from build123d import *

# Parameters (mm, degrees)
SKETCH2_R           = 14.2875
SKETCH2_R_2         = 3.556
BOSS_EXTRUDE1_DEPTH = 6.35


with BuildPart() as part:
    # Sketch2 → Boss-Extrude1 (new body)
    with BuildSketch(Plane(origin=(0, 0, 0), x_dir=(0, 0, -1), z_dir=(1, 0, 0))):
        with BuildLine():
            Line((-165.1, 34.925), (-80.596664787, 34.925))
            ThreePointArc((-80.596664787, 34.925), (-75.736585196, 33.958270063), (-71.616408666, 31.205256121))
            Line((-71.616408666, 31.205256121), (-20.205576272, -20.205576272))
            ThreePointArc((-20.205576272, -20.205576272), (-17.495774254, -22.592664922), (-14.50653847, -24.618914814))
            Line((-14.50653847, -24.618914814), (68.578013642, -73.575957012))
            ThreePointArc((68.578013642, -73.575957012), (78.454344121, -74.862548761), (86.221769537, -68.628422964))
            Line((86.221769537, -68.628422964), (133.536181692, 14.57458872))
            ThreePointArc((133.536181692, 14.57458872), (135.152284875, 21.909694343), (132.341634936, 28.875023547))
            Line((132.341634936, 28.875023547), (22.151863474, 164.100639036))
            ThreePointArc((22.151863474, 164.100639036), (-9.579695356, 172.971368128), (-28.575, 146.05))
            Line((-28.575, 146.05), (-33.807973228, 116.372334072))
            ThreePointArc((-33.807973228, 116.372334072), (-35.979801138, 112.610617786), (-40.061502459, 111.125))
            Line((-40.061502459, 111.125), (-88.9, 111.125))
            ThreePointArc((-88.9, 111.125), (-91.14506403, 110.19506403), (-92.075, 107.95))
            Line((-92.075, 107.95), (-92.075, 66.675))
            ThreePointArc((-92.075, 66.675), (-93.934871939, 62.184871939), (-98.425, 60.325))
            Line((-98.425, 60.325), (-165.1, 60.325))
            ThreePointArc((-165.1, 60.325), (-167.34506403, 59.39506403), (-168.275, 57.15))
            Line((-168.275, 57.15), (-168.275, 38.1))
            ThreePointArc((-168.275, 38.1), (-167.34506403, 35.85493597), (-165.1, 34.925))
        make_face()
        with Locations((0, 146.05)):
            Circle(SKETCH2_R, mode=Mode.SUBTRACT)
        Circle(SKETCH2_R, mode=Mode.SUBTRACT)
        with Locations((-53.975, 47.625)):
            Circle(SKETCH2_R_2, mode=Mode.SUBTRACT)
        with Locations((-79.375, 47.625)):
            Circle(SKETCH2_R_2, mode=Mode.SUBTRACT)
        with Locations((-104.775, 47.625)):
            Circle(SKETCH2_R_2, mode=Mode.SUBTRACT)
        with Locations((-130.175, 47.625)):
            Circle(SKETCH2_R_2, mode=Mode.SUBTRACT)
        with Locations((-155.575, 47.625)):
            Circle(SKETCH2_R_2, mode=Mode.SUBTRACT)
        with Locations((100.217738322, 10.071728166)):
            Circle(SKETCH2_R, mode=Mode.SUBTRACT)
        with Locations((-79.375, 73.025)):
            Circle(SKETCH2_R_2, mode=Mode.SUBTRACT)
        with Locations((-79.375, 98.425)):
            Circle(SKETCH2_R_2, mode=Mode.SUBTRACT)
        with BuildLine():
            Line((108.137843951, 33.631444269), (108.400752916, 34.22590106))
            ThreePointArc((108.400752916, 34.22590106), (111.416042328, 35.39192926), (112.582070528, 32.376639848))
            Line((112.582070528, 32.376639848), (112.319161563, 31.782183057))
            ThreePointArc((112.319161563, 31.782183057), (109.303872151, 30.616154857), (108.137843951, 33.631444269))
        make_face(mode=Mode.SUBTRACT)
        with BuildLine():
            Line((77.477027734, -4.031327927), (76.839593557, -4.822487627))
            ThreePointArc((76.839593557, -4.822487627), (76.346823941, -6.501290334), (77.185475983, -8.036823849))
            ThreePointArc((77.185475983, -8.036823849), (89.019434317, -15.248472927), (102.316672427, -19.151537226))
            ThreePointArc((102.316672427, -19.151537226), (104.016943026, -18.738886877), (104.927428038, -17.244826147))
            Line((104.927428038, -17.244826147), (105.083882379, -16.24094466))
            ThreePointArc((105.083882379, -16.24094466), (104.67123203, -14.54067406), (103.1771713, -13.630189049))
            ThreePointArc((103.1771713, -13.630189049), (91.279642465, -10.137973624), (80.691363956, -3.685445501))
            ThreePointArc((80.691363956, -3.685445501), (79.012561249, -3.192675886), (77.477027734, -4.031327927))
        make_face(mode=Mode.SUBTRACT)
    extrude(amount=BOSS_EXTRUDE1_DEPTH)


solid = part.part
Geometry: final body of the model. Coordinates: model frame, mm. A direction names the side the tool comes from. Give positions to 0.01 mm unless a question says otherwise; leave off trailing zeros. Order: outer loops, then holes, each group sorted by start corner. A loop starts at its lowest first (then second) coordinate and runs counter-clockwise, first axis right, second up. Notation, with made-up numbers: (15, -23.75) -> (34, -23.75) arc R20 ccw to (34, 15.25) -> close; hole circle Ø10 at (18, 61.5). An arc over 180 degrees is marked (long way). Write each question's results on one line, items separated by ' | '.
1) Cut plane A-A (y = 0). Output: boundary loops of the cut face in (x, z), and give its area (3 significant figures).
Geometry says:
outline: (0, -125.25) -> (6.35, -125.25) -> (6.35, -110.35) -> (0, -110.35) -> close; (0, -90.08) -> (6.35, -90.08) -> (6.35, -14.29) -> (0, -14.29) -> close; (0, 14.29) -> (6.35, 14.29) -> (6.35, 40.41) -> (0, 40.41) -> close | area: 742 mm²
2) Cut plane B-B (z = 0). Give the number of separate pieces and of enclosed holes in the cut face, and give its area (3 significant figures).
Geometry says:
separate pieces: 3 | enclosed holes: 0 | area: 957 mm²
3) Draft query along Z for faces 6 (the face through (3.13, 95.54, -78.02)), 7 (the face through (3, 111.125, 64)), 8 (the face through (3.13, 46.26, 76.09)). Return one class per face: released by +Z, released by -Z, zero draft, split by the parting line, or undercut.
Geometry says:
face 6: released by -Z | face 7: zero draft | face 8: undercut
4) Cut plane C-C (y = 137). Output: boundary loops of the cut face in (x, z), and give its area (3 significant figures).
Geometry says:
outline: (0, -44.24) -> (6.35, -44.24) -> (6.35, -11.06) -> (0, -11.06) -> close; (0, 11.06) -> (6.35, 11.06) -> (6.35, 30.17) -> (0, 30.17) -> close | area: 332 mm²
5) Line query: line 1 along Y through (x, z) = (2.25, -9.5); line 2 along Y through (x, z) = (2, 0) (1 decimal); line 3 along Y through (x, z) = (4.5, 114) (3 decimals). Output: solid intervals per line, ascending.
Geometry says:
line 1: y = -38.76 to -10.67, 10.67 to 135.38, 156.72 to 173 | line 2: y = -33.2 to -14.3, 14.3 to 131.8, 160.3 to 174.6 | line 3: y = 34.925 to 60.325
6) First-contact query: pin 1 Ø3 at (x, z) = (2, 70) entering from +Y (3 decimals); pin 2 Ø1.5 at (x, y) = (3.5, 73.5) entering from -Z; pin 3 Ø1.9 at (x, z) = (4, 102.5) entering from -Y (3 decimals). Flat tips, straight axial feed; report the tip coordinate or a pass-through.
Geometry says:
pin 1: stops at y = 111.125 | pin 2: stops at z = -96.59 | pin 3: stops at y = 34.925
7) Set-up query: faces 1 (the face through (3, 34.925, 123)), 2 (the face through (3, 88, 92.075)), 3 (the face through (3.13, -10.21, -91.44)), 4 (the face through (3.13, -74.9, -78.32)), 5 (the face through (6.35, 51, -15)). Return all of +Z, -Z, +X, -X, +Y, -Y with unobstructed straight access to the full face (end or side cutting, diameter ignored); none if empty.
Geometry says:
face 1: +Z, +X, -X, -Y | face 2: +Z, +X, -X, +Y | face 3: +X, -X | face 4: +X, -X, -Y | face 5: +Z, -Z, +X, +Y, -Y
